Verification items for the finished model (mm, model axes). Face numbers are marked on the shaded views. A direction names the side the tool comes from. Round coordinates to 2 decimals unless told otherwise and drop trailing zeros. Write each loop counter-clockwise with the first axis right and the second up, starting at its lowest first coordinate (ties: lowest second). Pieces come first, ordered by that corner, then holes. Notation, with made-up numbers: (-24.75, -23.75) -> (-19.75, -23.75) arc R17 ccw to (-19.75, -13.75) -> close; hole circle Ø1 at (5.25, 88). An arc over 180 degrees is marked (long way). Answer as a JSON object with one key per item and string values. Group by question number.
(1) Scan lines: L1, parallel to X at y = -6.9, z = -1; L2, parallel to Y at x = 13, z = 2.5; L3, parallel to Y at x = -13, z = 6. Record each from-to range of solid material in increasing order. Write a range as from..to.
(2) Sectioned sample at C-C on y = 4.5. Record the cut outline in (x, z), and give its area (3 significant figures).
(3) Gauge pin test, flat ends, axial feed: pin 1 Ø4 at (x, z) = (-4.5, -7.5) entering from +Y; pin 2 Ø1.8 at (x, y) = (-12.5, 5) entering from -Z; pin 3 Ø0.8 at (x, z) = (0.5, 7.5) entering from +Y. Record the tip position at first contact, or that the pin passes through.
(4) Draft check along Z on the marked faces 4, 5 and 6. Enter one of: released by +Z, released by -Z, zero draft, split by the parting line, or undercut.
(5) Sectioned sample at B-B on y = -5.25. Record the cut outline in (x, z), and give its area (3 significant figures).
(6) Set-up check for the marked faces 1, 2 and 3: record each of +Z, -Z, +X, -X, +Y, -Y from which the full face is reachable in a straight line by a thin tool's end or side.
(7) Sectioned sample at D-D on x = 0. Record the cut outline in (y, z).
```python
from build123d import *

# Parameters (mm, degrees)
SKETCH1_W           = 35
SKETCH1_H           = 18
BOSS_EXTRUDE1_DEPTH = 8
SKETCH4_W           = 18
SKETCH4_H           = 10
CUT_EXTRUDE3_DEPTH  = 1
CUT_EXTRUDE2_REACH  = 23.243
SKETCH3_R           = 1.65
SKETCH5_R           = 3
CUT_EXTRUDE4_DEPTH  = 4
SKETCH6_W           = 35
SKETCH6_H           = 7.5
BOSS_EXTRUDE2_DEPTH = 10
SKETCH7_R           = 8
CUT_EXTRUDE5_DEPTH  = 4.8
FILLET1_R           = 2.5


with BuildPart() as part:
    # Sketch1 → Boss-Extrude1 (new body)
    with BuildSketch(Plane.XY):
        Rectangle(SKETCH1_W, SKETCH1_H)
    extrude(amount=BOSS_EXTRUDE1_DEPTH)

    # Sketch4 → Cut-Extrude3 (cut)
    with BuildSketch(Plane.XY.offset(8)):
        with Locations((0, 4)):
            Rectangle(SKETCH4_W, SKETCH4_H)
    extrude(amount=-CUT_EXTRUDE3_DEPTH, mode=Mode.SUBTRACT)

    # Sketch3 → Cut-Extrude2 (cut, up to next)
    with BuildSketch(Plane(origin=(0, 0, 0), x_dir=(-1, 0, 0), z_dir=(0, 0, -1)), mode=Mode.PRIVATE) as cut_extrude2_sk1:
        with Locations((-13, 4)):
            Circle(SKETCH3_R)
    cut_extrude2_tool1 = extrude(cut_extrude2_sk1.sketch, amount=-CUT_EXTRUDE2_REACH, mode=Mode.PRIVATE) & part.part
    # Sketch3 → Cut-Extrude2 (cut, up to next)
    with BuildSketch(Plane(origin=(0, 0, 0), x_dir=(-1, 0, 0), z_dir=(0, 0, -1)), mode=Mode.PRIVATE) as cut_extrude2_sk2:
        with Locations((13, 4)):
            Circle(SKETCH3_R)
    cut_extrude2_tool2 = extrude(cut_extrude2_sk2.sketch, amount=-CUT_EXTRUDE2_REACH, mode=Mode.PRIVATE) & part.part
    add(cut_extrude2_tool1.solids().sort_by_distance((13, 4, 0))[0], mode=Mode.SUBTRACT)
    add(cut_extrude2_tool2.solids().sort_by_distance((-13, 4, 0))[0], mode=Mode.SUBTRACT)

    # Sketch5 → Cut-Extrude4 (cut)
    with BuildSketch(Plane(origin=(0, 0, 0), x_dir=(-1, 0, 0), z_dir=(0, 0, -1))):
        with Locations((-13, 4)):
            Circle(SKETCH5_R)
        with Locations((13, 4)):
            Circle(SKETCH5_R)
    extrude(amount=-CUT_EXTRUDE4_DEPTH, mode=Mode.SUBTRACT)

    # Sketch6 → Boss-Extrude2 (add)
    with BuildSketch(Plane.XY):
        with Locations((0, -5.25)):
            Rectangle(SKETCH6_W, SKETCH6_H)
    extrude(amount=-BOSS_EXTRUDE2_DEPTH)

    # Sketch7 → Cut-Extrude5 (cut)
    with BuildSketch(Plane(origin=(0, -9, 0), x_dir=(-1, 0, 0), z_dir=(0, -1, 0))):
        with Locations(Location((0, 1, 0), (0, 0, 90))):
            Circle(SKETCH7_R)
    extrude(amount=-CUT_EXTRUDE5_DEPTH, mode=Mode.SUBTRACT)

    # Fillet1
    fillet1_edges = [part.edges().sort_by_distance(p)[0] for p in [
        (17.5, -5.25, -10),
        (-17.5, -5.25, -10),
        (0, -1.5, 0),
    ]]
    fillet(fillet1_edges, radius=FILLET1_R - 0.0001)  # a hair under: the kernel refuses the full size


solid = part.part
```
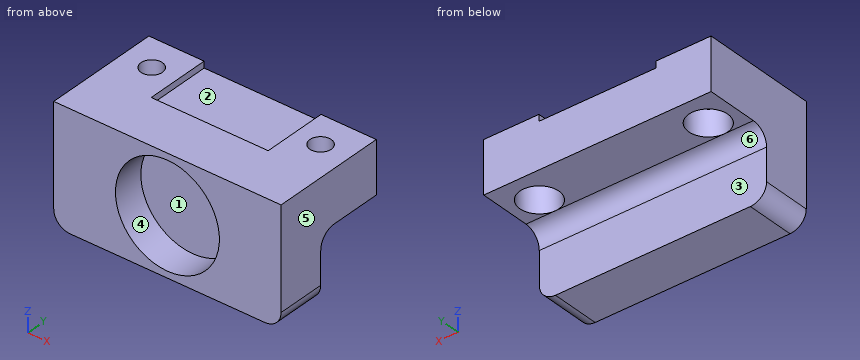
Computed values:
{
 "1": {"L1": "-17.5..-8, 8..17.5", "L2": "-9..1, 7..9", "L3": "-9..2.35, 5.65..9"},
 "2": {"outline": "(-17.5, 0) -> (-15.96, 0) -> (-15.96, 4) -> (-14.57, 4) -> (-14.57, 8) -> (-17.5, 8) -> close; (-11.43, 4) -> (-10.04, 4) -> (-10.04, 0) -> (10.04, 0) -> (10.04, 4) -> (11.43, 4) -> (11.43, 8) -> (9, 8) -> (9, 7) -> (-9, 7) -> (-9, 8) -> (-11.43, 8) -> close; (14.57, 4) -> (15.96, 4) -> (15.96, 0) -> (17.5, 0) -> (17.5, 8) -> (14.57, 8) -> close", "area": "190 mm2"},
 "3": {"pin 1": "y = -1.5", "pin 2": "z = 4", "pin 3": "y = -1"},
 "4": {"face 4": "undercut", "face 5": "zero draft", "face 6": "released by -Z"},
 "5": {"outline": "(-17.5, -7.5) arc R2.5 ccw to (-15, -10) -> (15, -10) arc R2.5 ccw to (17.5, -7.5) -> (17.5, 8) -> (-17.5, 8) -> close; hole circle Ø16 at (0, -1)", "area": "426 mm2"},
 "6": {"face 1": "-Y", "face 2": "+Z, +Y", "face 3": "-Z, +X, -X, +Y"},
 "7": {"outline": "(-9, -10) -> (-1.5, -10) -> (-1.5, -2.5) arc R2.5 cw to (1, 0) -> (9, 0) -> (9, 7) -> (-1, 7) -> (-1, 8) -> (-9, 8) -> (-9, 7) -> (-4.2, 7) -> (-4.2, -9) -> (-9, -9) -> close"}
}
